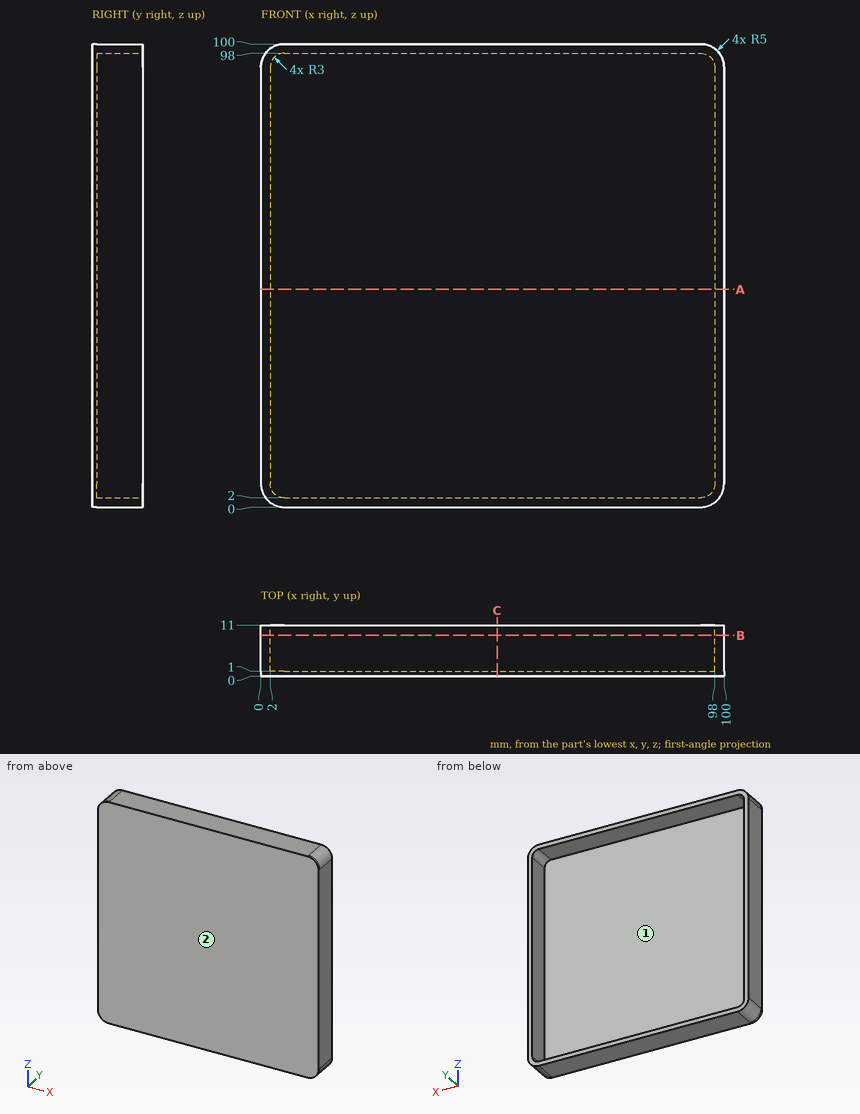
Source: three-view drawing plus pictorial views. Frame: mm from the lowest corner of the part. Coordinates: 2 decimals unless noted, no trailing zeros. Order: outer loops, then holes, each group sorted by start corner. A loop starts at its lowest first (then second) coordinate and runs counter-clockwise, first axis right, second up. Notation, with made-up numbers: M -33.5,40.5 L -26.5,40.5 A24 ccw -26.5,69.5 Z; hole C -38,64.5 d8. An arc over 180 degrees is marked long. One line per question, with ' | ' between items. Start each with the question number.
Item 1: Draft query along X for the marked faces 1 and 2. Return one class per face: released by +X, released by -X, zero draft, split by the parting line, or undercut.
Item 2: Pin query (flat end, axial travel): pin 1 Ø4 at (x, z) = (27, 73) entering from +Y. Return the tip coordinate at first contact, or that it passes through.
Item 3: Cut plane B-B, the plane y = 8.75. Return the cut outline in (x, z), then the cut area to 3 significant figures.
Item 4: Cut plane C-C, the plane x = 51. Return the cut outline in (y, z), then the cut area to 3 significant figures.
Item 5: Cut plane A-A, the plane z = 47. Return the cut outline in (x, y).
Item 6: Ray query, probe 1 along Z at (x, y) = (62, 8.75); probe 2 along Y at (x, z) = (38, 46). Return the intervals inside material, ascending. Write a range as [from, to].
A:
1) face 1: undercut | face 2: zero draft
2) pin 1: stops at y = 1
3) outline: M 0,5 A5 ccw 5,0 L 95,0 A5 ccw 100,5 L 100,95 A5 ccw 95,100 L 5,100 A5 ccw 0,95 Z; hole M 2,5 A3 ccw 5,2 L 95,2 A3 ccw 98,5 L 98,95 A3 ccw 95,98 L 5,98 A3 ccw 2,95 Z | area: 770 mm2
4) outline: M 0,0 L 11,0 L 11,2 L 1,2 L 1,98 L 11,98 L 11,100 L 0,100 Z | area: 140 mm2
5) outline: M 0,0 L 100,0 L 100,11 L 98,11 L 98,1 L 2,1 L 2,11 L 0,11 Z
6) probe 1: z = [0, 2], [98, 100] | probe 2: y = [0, 1]
